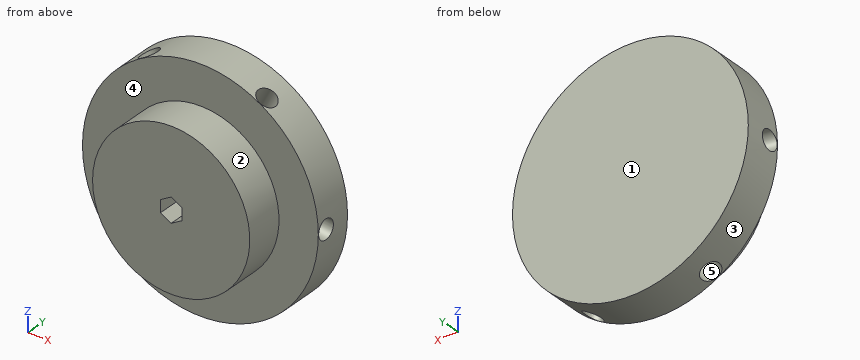
Autodesk Inventor part; units mm, degrees
ref_plane "作業平面2" through (0, 8.7, 3) normal (-0.9877, -0.1564, 0) x (0, 0, 1)
ref_plane "YZ Plane" through (0, 0, 0) normal (1, 0, 0) x (0, 1, 0)
ref_plane "XZ Plane" through (0, 0, 0) normal (0, 1, 0) x (-1, 0, 0)
sketch "スケッチ1" plane through (0, 0, 0) normal (0, 1, 0) x (-1, 0, 0)
  circle A0 centre (0, 0) radius 10
  dimension "d0" = 20
extrude "押し出し1" add sketch "スケッチ1" along normal blind 5
sketch "スケッチ2" plane through (0, 5, 0) normal (0, 1, 0) x (1, 0, 0)
  circle A0 centre (0, 0) radius 15
  dimension "dia_rod_base" = 30
extrude "押し出し2" add sketch "スケッチ2" along normal blind 5
sketch "スケッチ5" plane through (0, 0, 0) normal (0, -1, 0) x (1, 0, 0)
  line L0 (0, 1.5588) -> (1.35, 0.7794)
  line L1 (1.35, 0.7794) -> (1.35, -0.7794)
  line L2 (1.35, -0.7794) -> (0, -1.5588)
  line L3 (0, -1.5588) -> (-1.35, -0.7794)
  line L4 (-1.35, -0.7794) -> (-1.35, 0.7794)
  line L5 (-1.35, 0.7794) -> (0, 1.5588)
  point P0 (0, 0)
  point P1 (0, 0)
  dimension "d14" = 2.7
extrude "押し出し3" cut sketch "スケッチ5" against normal blind 5
ref_plane "作業平面1" through (0, 0, 3) normal (0, 0, 1) x (1, 0, 0)
sketch "スケッチ10" plane through (0, 0, 3) normal (0, 0, 1) x (1, 0, 0)
  line L0 (15, 10) -> (-15, 10)
  line L1 (15, 10) -> (-15, 10)
  line L2 (15, 5) -> (-15.1085, 12.4268)
  line L3 (15, 5) -> (15, 10)
  line L4 (15, 5) -> (-15.1085, 12.4268)
  point P0 (0, 0)
  point P1 (0, 8.7)
  point P2 (0, 10)
  point P3 (-0.0543, 8.7134)
  dimension "d30" = 15
  dimension "d37" = 1.3
ref_plane "作業平面2" through (0, 8.7, 3) normal (-0.9877, -0.1564, 0) x (0, 0, 1)
sketch "スケッチ11" plane through (0, 8.7, 3) normal (-0.9877, -0.1564, 0) x (0, 0, 1)
  circle A0 centre (-3, 0) radius 1.25
  line L0 (-18, -3.6544) -> (-18, 1.284)
  line L1 (12, -3.6544) -> (12, 1.284)
  line L2 (-24, 0) -> (18, 0)
  point P0 (-3, -8.5929)
  dimension "d32" = 2.5
  dimension "d33" = 15
extrude "押し出し6" cut sketch "スケッチ11" along normal through all
pattern_circular "円形状パターン2" count 6 over 360 about axis through (0, 5, 0) along (0, 1, 0) of "押し出し6"
properties part number "exp_tire_6rod_lower_rev0"
Check sheet for the modelled part. Datum: model origin and axes. Units: mm. Face numbers are marked on the shaded views. A direction names the side the tool comes from. Give positions to 0.01 mm unless a question says otherwise; leave off trailing zeros. Order: outer loops, then holes, each group sorted by start corner. A loop starts at its lowest first (then second) coordinate and runs counter-clockwise, first axis right, second up. Notation, with made-up numbers: M 17,19.5 L 64,19.5 A13 cw 64,27.5 Z; hole C -39,-20.5 d3. An arc over 180 degrees is marked long. Answer as CSV lines item,"result". Start each with the question number.
Item 1: Tool access check on the marked faces 1 and 2. Record the directions out of +Z, -Z, +X, -X, +Y, -Y that give a thin tool (end or side, any length) a straight path to the whole face; none if there is none.
Item 2: Thickness scan on line 1 (X direction, y = 7, z = 5); line 2 (Z direction, x = -2.5, y = 8.75); line 3 (Y direction, x = -7, z = 8). Record the ranges inside material, lowest first. Write a range as [from, to].
Item 3: Cross-section at A-A on y = 3.25. Enter the section's corners in (x, z), plus the area to 3 significant figures.
Item 4: Cross-section at B-B on z = 3. State how many separate pieces and enclosed holes the cut face has, plus the area to 3 significant figures.
Item 5: Mould release check, pull along Z, two halves, no side actions. Record for the marked faces 3, 4 and 5: +Z half, -Z half, draft (parallel to the pull), parting line (faces both ways), or undercut.
Item 6: Gauge pin test, flat ends, axial feed: P1, Ø1.5, axis at y = 8, z = -11.5, coming from the -X side; P2, Ø0.8, axis at y = 3.5, z = 0, coming from the -X side; P3, Ø1, axis at x = -8, y = 2, coming from the +Z side. Record the tip position at first contact, or that the pin passes through.
Established:
1,face 1,"+Z, -Z, +X, -X, +Y"
1,face 2,"-Y"
2,line 1,"x = [-14.14, -4.1], [-1.84, 1.84], [4.1, 14.14]"
2,line 2,"z = [-14.79, -5.76], [-2.06, -1.17], [1.17, 2.06], [5.76, 14.79]"
2,line 3,"y = [5, 10]"
3,outline,"C 0,0 d20; hole M -1.35,-0.78 L 0,-1.56 L 1.35,-0.78 L 1.35,0.78 L 0,1.56 L -1.35,0.78 Z"
3,area,"308 mm^2"
4,separate pieces,"1"
4,enclosed holes,"2"
4,area,"231 mm^2"
5,face 3,"parting line"
5,face 4,"draft"
5,face 5,"undercut"
6,P1,"stops at x = -10.46"
6,P2,"stops at x = -10"
6,P3,"stops at z = 6.61"
